Source: three-view drawing plus pictorial views. Frame: mm from the lowest corner of the part. A direction names the side the tool comes from. Give positions to 0.01 mm unless a question says otherwise; leave off trailing zeros. Loops run counter-clockwise (first coordinate to the right, second up) from the corner with the lowest first, then second, coordinate; pieces in that order, holes last. Notation, with made-up numbers: (6.5, -32) -> (39.5, -32) arc R19 cw to (39.5, -22) -> close; hole circle Ø4 at (89.25, 26). An arc over 180 degrees is marked (long way). Answer as a JSON object with one key per item and string values. Group by question number.
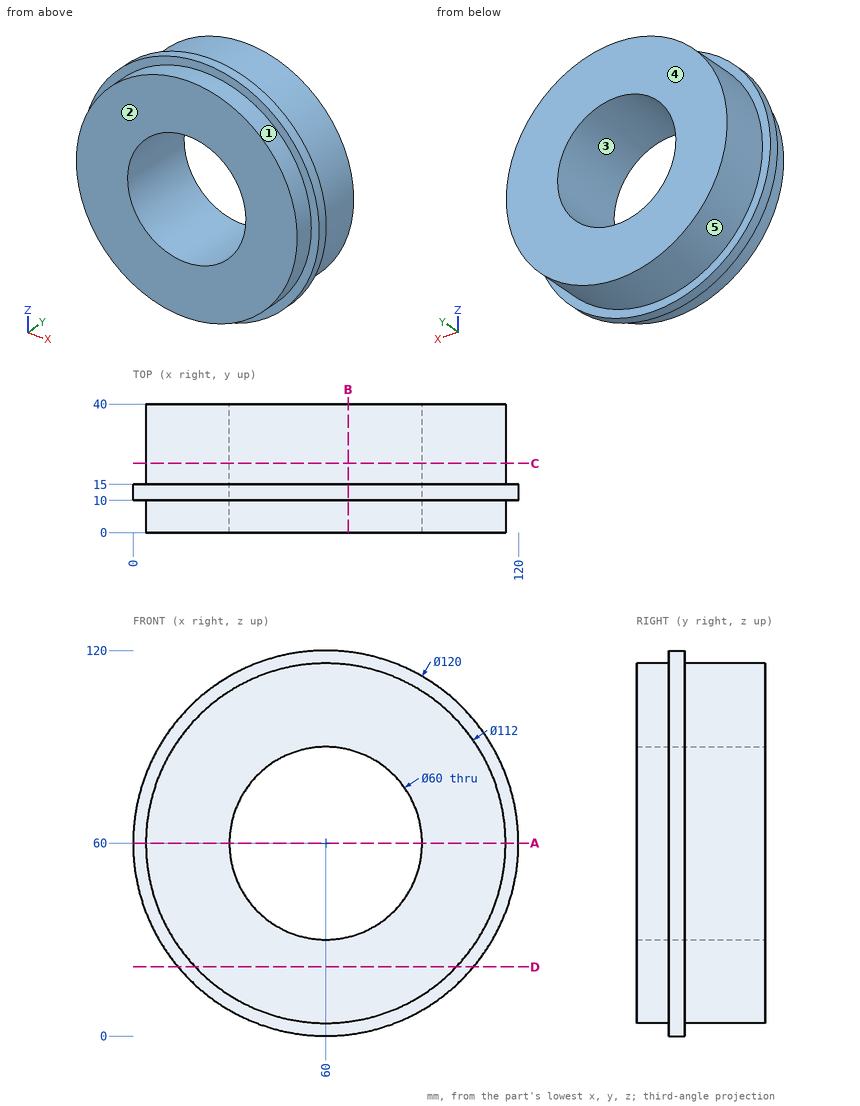
Q1. Section D-D on z = 21.5. Return the cut outline in (x, y), then the cut area to 3 significant figures.
Q2. Ray query, probe 1 along Z at (x, y) = (60, 19); probe 2 along Z at (x, y) = (60, 10.5). Return the intervals inside material, ascending.
Q3. Pin query (flat end, axial travel): pin 1 Ø6 at (y, z) = (19.5, 106) entering from -X; pin 2 Ø10 at (x, z) = (26.5, 97.5) entering from -Y; pin 3 Ø3 at (x, y) = (84, 21.5) entering from +Z; pin 4 Ø3 at (y, z) = (21.5, 98.5) entering from -X. Return the tip coordinate at first contact, or that it passes through.
Q4. Section C-C on y = 21.5. Return the cut outline in (x, z).
Q5. Set-up query: the marked faces 1 and 2. Return all of +Z, -Z, +X, -X, +Y, -Y with unobstructed straight access to the full face (end or side cutting, diameter ignored); none if empty.
Q6. Section A-A on z = 60. Return the cut outline in (x, y), then the cut area to 3 significant figures.
Q7. Section B-B on x = 67. Return the cut outline in (y, z).
Q8. Pull-direction query (Z, two-part tool) for the marked faces 3, 4 and 5; classes: +Z half, -Z half, draft (parallel to the pull), parting line (faces both ways), or undercut.
Numbers:
{
 "1": {"outline": "(13.98, 10) -> (19.33, 10) -> (19.33, 0) -> (100.67, 0) -> (100.67, 10) -> (106.02, 10) -> (106.02, 15) -> (100.67, 15) -> (100.67, 40) -> (19.33, 40) -> (19.33, 15) -> (13.98, 15) -> close", "area": "3,310 mm²"},
 "2": {"probe 1": "z = 4 to 30, 90 to 116", "probe 2": "z = 0 to 30, 90 to 120"},
 "3": {"pin 1": "stops at x = 24.13", "pin 2": "stops at y = 0", "pin 3": "stops at z = 111.28", "pin 4": "stops at x = 17.96"},
 "4": {"outline": "circle Ø112 at (60, 60); hole circle Ø60 at (60, 60)"},
 "5": {"face 1": "-Y", "face 2": "+Z, -Z, +X, -X, -Y"},
 "6": {"outline": "(0, 10) -> (4, 10) -> (4, 0) -> (30, 0) -> (30, 40) -> (4, 40) -> (4, 15) -> (0, 15) -> close; (90, 0) -> (116, 0) -> (116, 10) -> (120, 10) -> (120, 15) -> (116, 15) -> (116, 40) -> (90, 40) -> close", "area": "2,120 mm²"},
 "7": {"outline": "(0, 4.44) -> (10, 4.44) -> (10, 0.41) -> (15, 0.41) -> (15, 4.44) -> (40, 4.44) -> (40, 30.83) -> (0, 30.83) -> close; (0, 89.17) -> (40, 89.17) -> (40, 115.56) -> (15, 115.56) -> (15, 119.59) -> (10, 119.59) -> (10, 115.56) -> (0, 115.56) -> close"},
 "8": {"face 3": "undercut", "face 4": "draft", "face 5": "parting line"}
}
